Job drawing, mm, ordinate dimensions from the low corner. One solid piece. A direction names the side the tool comes from. Coordinates: 2 decimals unless noted, no trailing zeros. Order: outer loops, then holes, each group sorted by start corner. A loop starts at its lowest first (then second) coordinate and runs counter-clockwise, first axis right, second up. Notation, with made-up numbers: (64.25, 12.25) - (69.25, 12.25) arc R22 cw to (69.25, 20.25) - close; hole circle Ø8 at (32.25, 46). An arc over 180 degrees is marked (long way). Return JSON: item names as keys, results as strings.
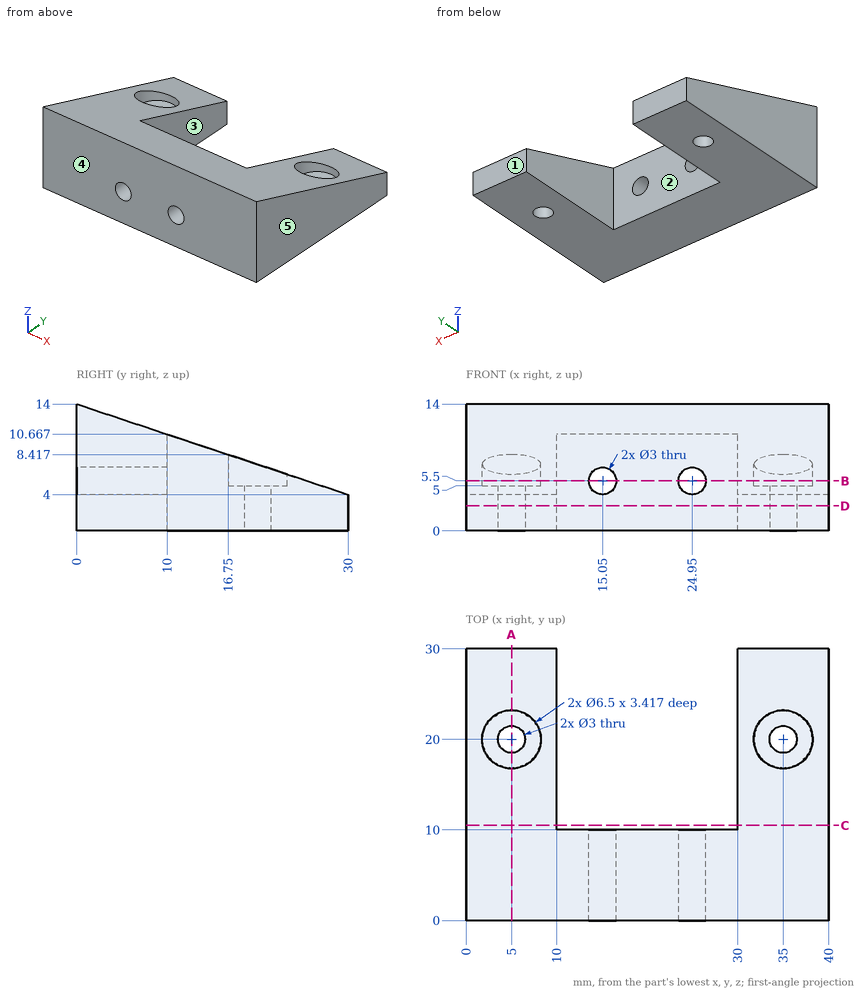
1. Cut at B-B on z = 5.5. Give the cut face in (x, y).
Check values:
{"outline": "(0, 0) - (13.55, 0) - (13.55, 10) - (10, 10) - (10, 25.5) - (0, 25.5) - close; (16.55, 0) - (23.45, 0) - (23.45, 10) - (16.55, 10) - close; (26.45, 0) - (40, 0) - (40, 25.5) - (30, 25.5) - (30, 10) - (26.45, 10) - close; hole circle Ø6.5 at (5, 20); hole circle Ø6.5 at (35, 20)"}
2. Cut at C-C on y = 10.5. Give the cut face in (x, z).
Check values:
{"outline": "(0, 0) - (10, 0) - (10, 10.5) - (0, 10.5) - close; (30, 0) - (40, 0) - (40, 10.5) - (30, 10.5) - close"}
3. Cut at A-A on x = 5. Give the cut face in (y, z).
Check values:
{"outline": "(0, 0) - (18.5, 0) - (18.5, 5) - (16.75, 5) - (16.75, 8.42) - (0, 14) - close; (21.5, 0) - (30, 0) - (30, 4) - (23.25, 6.25) - (23.25, 5) - (21.5, 5) - close"}
4. Drop flat-ended pins along their axis: pin 1 (1.8 mm diameter, centred on x = 24.95, z = 5.5, fed in from +Y); pin 2 (5 mm diameter, centred on x = 5, y = 20, fed in from +Z); pin 3 (7.5 mm diameter, centred on x = 5, y = 20, fed in from +Z); pin 4 (3.5 mm diameter, centred on x = 15.05, z = 5.5, fed in from +Y). Give the stop position or say it passes through.
Check values:
{"pin 1": "through", "pin 2": "z = 5", "pin 3": "z = 8.58", "pin 4": "y = 10"}
5. Probe L1, parallel to X at y = 4.25, z = 5.5; L2, parallel to X at y = 20, z = 7; L3, parallel to X at y = 16, z = 1. List the from-to ranges inside material, lowest first.
Check values:
{"L1": "0 to 13.55, 16.55 to 23.45, 26.45 to 40", "L2": "0 to 1.75, 8.25 to 10, 30 to 31.75, 38.25 to 40", "L3": "0 to 10, 30 to 40"}
6. Tool access for the marked faces 1 and 2: list every direction of +Z, -Z, +X, -X, +Y, -Y with a clear straight run to the whole face (end or side of a thin tool).
Check values:
{"face 1": "+Z, -Z, +X, -X, +Y", "face 2": "+Z, -Z, +Y"}
7. Cut at D-D on z = 2.75. Give the cut face in (x, y).
Check values:
{"outline": "(0, 0) - (40, 0) - (40, 30) - (30, 30) - (30, 10) - (10, 10) - (10, 30) - (0, 30) - close; hole circle Ø3 at (5, 20); hole circle Ø3 at (35, 20)"}
8. Mould opens along X. For the marked faces 3, 4 and 5 say: pulls with the +X half, pulls with the -X half, needs draft (parallel to the pull), parting line crosses it, or undercut.
Check values:
{"face 3": "undercut", "face 4": "needs draft", "face 5": "pulls with the +X half"}
